from build123d import *

# Parameters (mm, degrees)
SKETCH_1_W                 = 160
SKETCH_1_H                 = 250
EXTRUDE_271_DEPTH          = 10
SKETCH_6_W                 = 45
SKETCH_6_H                 = 130
EXTRUDE_648_DEPTH          = 3
HOLE_WIZARD_M3_D           = 3.4
HOLE_WIZARD_M3_CSINK_D     = 6.3
HOLE_WIZARD_M3_CSINK_ANGLE = 90
HOLE_WIZARD_M5_D           = 5.5
HOLE_WIZARD_M5_CSINK_D     = 10.4
HOLE_WIZARD_M5_CSINK_ANGLE = 90


with BuildPart() as part:
    # Эскиз1 → Extrude 271 (new body)
    with BuildSketch(Plane.XY):
        Rectangle(SKETCH_1_W, SKETCH_1_H)
    extrude(amount=EXTRUDE_271_DEPTH)

    # Эскиз6 → Extrude 648 (add)
    with BuildSketch(Plane(origin=(0, 0, 0), x_dir=(-1, 0, 0), z_dir=(0, 0, -1))):
        with Locations((-57.5, 60)):
            Rectangle(SKETCH_6_W, SKETCH_6_H)
        with Locations((57.5, 60)):
            Rectangle(SKETCH_6_W, SKETCH_6_H)
    extrude(amount=EXTRUDE_648_DEPTH)

    # Каретки-M3 (through all)
    with Locations(Plane.XY.offset(10)):
        with Locations((-67.5, 107.5), (-42.5, 107.5), (-42.5, 82.5), (-67.5, 82.5), (42.5, 107.5), (67.5, 107.5), (67.5, 82.5), (42.5, 82.5), (-67.5, 42.5), (-42.5, 42.5), (-42.5, 17.5), (-67.5, 17.5), (42.5, 42.5), (67.5, 42.5), (67.5, 17.5), (42.5, 17.5)):
            CounterSinkHole(HOLE_WIZARD_M3_D / 2, HOLE_WIZARD_M3_CSINK_D / 2, counter_sink_angle=HOLE_WIZARD_M3_CSINK_ANGLE)

    # Гайка ШВП - M5 (through all)
    with Locations(Plane.XY.offset(10)):
        with Locations((-16, 40), (16, 40)):
            CounterSinkHole(HOLE_WIZARD_M5_D / 2, HOLE_WIZARD_M5_CSINK_D / 2, counter_sink_angle=HOLE_WIZARD_M5_CSINK_ANGLE)


solid = part.part
Geometry check sheet. Reference: the model listing, model coordinates, mm. Give positions to 0.01 mm unless a question says otherwise; leave off trailing zeros. Loops run counter-clockwise (first coordinate to the right, second up) from the corner with the lowest first, then second, coordinate; pieces in that order, holes last. Notation, with made-up numbers: (88.25, 85) -> (98.25, 85) arc R21 ccw to (98.25, 106) -> close; hole circle Ø11 at (62.5, 56.25). An arc over 180 degrees is marked (long way). Answer in a Markdown table with one row per item. Add a question column.
1) Cross-section at B-B on y = 23.5. Record the boundary of the cut face in (x, z), and give its area (3 significant figures).
2) Cross-section at C-C on y = -70.5. Record the boundary of the cut face in (x, z).
3) Draft check along X on faces 1 (the face through (80, -2, 4)), 2 (the face through (14.46, 42.42, 7.67)), 3 (the face through (-1, -26, 0)), 4 (the face through (-1, -125, 5)). Enter one of: pulls with the +X half, pulls with the -X half, needs draft (parallel to the pull), parting line crosses it, or undercut.
4) Gauge pin test, flat ends, axial feed: P1, Ø5.5, axis at x = 42.5, y = 82.5, coming from the +Z side; P2, Ø4, axis at x = -42.5, y = 42.5, coming from the +Z side; P3, Ø7, axis at x = 16, y = 40, coming from the -Z side. Record the tip position at first contact, or that the pin passes through.
5) Cross-section at A-A on x = 16. Record the boundary of the cut face in (y, z).
6) Material ranges on probe 1 along Y at (x, z) = (42.5, 2); probe 2 along Y at (x, z) = (67.5, -0.25); probe 3 along X at (y, z) = (82.5, 2), recorded low to high. Write a range as from..to.
Outcome:
| question | item | result |
|---|---|---|
| 1 | outline | (-80, -3) -> (-35, -3) -> (-35, 0) -> (35, 0) -> (35, -3) -> (80, -3) -> (80, 10) -> (-80, 10) -> close |
| 1 | area | 1,870 mm^2 |
| 2 | outline | (-80, 0) -> (80, 0) -> (80, 10) -> (-80, 10) -> close |
| 3 | face 1 | pulls with the +X half |
| 3 | face 2 | undercut |
| 3 | face 3 | undercut |
| 3 | face 4 | needs draft |
| 4 | P1 | stops at z = 9.6 |
| 4 | P2 | stops at z = 8.85 |
| 4 | P3 | stops at z = 0 |
| 5 | outline | (-125, 0) -> (37.25, 0) -> (37.25, 7.55) -> (34.8, 10) -> (-125, 10) -> close; (42.75, 0) -> (125, 0) -> (125, 10) -> (45.2, 10) -> (42.75, 7.55) -> close |
| 6 | probe 1 | y = -125..15.8, 19.2..40.8, 44.2..80.8, 84.2..105.8, 109.2..125 |
| 6 | probe 2 | y = -5..15.8, 19.2..40.8, 44.2..80.8, 84.2..105.8, 109.2..125 |
| 6 | probe 3 | x = -80..-69.2, -65.8..-44.2, -40.8..40.8, 44.2..65.8, 69.2..80 |
